Input: part model. Units: mm. Frame: model coordinates. Give positions to 0.01 mm unless a question says otherwise; leave off trailing zeros. Loops run counter-clockwise (first coordinate to the right, second up) from the corner with the lowest first, then second, coordinate; pieces in that order, holes last. Notation, with made-up numbers: M 67.25,60 L 111.25,60 A10 cw 111.25,64 Z; hole C -38.5,-6.75 d9. An arc over 180 degrees is marked long. Answer as a JSON object with one key per item and string values. Group by question number.
1) Section query C-C on z = 172.4. Return loops of the section in (x, y).
2) Section query A-A on z = -192.4. Return loops of the section in (x, y).
3) First-contact query: P1, Ø9.5, axis at y = -29.33, z = 172.4, coming from the +X side. Flat tip, straight axial feed; report the tip coordinate or a pass-through.
4) Section query B-B on x = 1. Return loops of the section in (y, z).
5) Ray query, L1, parallel to Z at x = 15.5, y = -36.75; L2, parallel to Z at x = 19, y = -33; L3, parallel to Z at x = 27.5, y = -24.5. Return the intervals inside material, ascending.
from build123d import *

# Parameters (mm, degrees)
SKETCH1_W           = 35
SKETCH1_H           = 30
BOSS_EXTRUDE1_DEPTH = 202.4
SKETCH4_R           = 6
CUT_EXTRUDE1_DEPTH  = 211.132863092
SKETCH5_R           = 6
CUT_EXTRUDE2_DEPTH  = 208.132591643
CHAMFER1_SIZE       = 0.3


with BuildPart() as part:
    # Sketch1 → Boss-Extrude1 (new, symmetric)
    with BuildSketch(Plane.XY):
        with Locations((14.720343273, -29.328998989)):
            Rectangle(SKETCH1_W, SKETCH1_H)
    extrude(amount=BOSS_EXTRUDE1_DEPTH, both=True)

    # Sketch4 → Cut-Extrude1 (cut, through all)
    with BuildSketch(Plane.ZY.offset(2.779656727)):
        with Locations(Location((172.4, -29.328998989, 0), (0, 0, 270))):
            Circle(SKETCH4_R)
        with Locations(Location((62.4, -29.328998989, 0), (0, 0, 270))):
            Circle(SKETCH4_R)
        with Locations(Location((117.4, -29.328998989, 0), (0, 0, 270))):
            Circle(SKETCH4_R)
    extrude(amount=-CUT_EXTRUDE1_DEPTH, mode=Mode.SUBTRACT)

    # Sketch5 → Cut-Extrude2 (cut, through all)
    with BuildSketch(Plane(origin=(0, -14.328998989, 0), x_dir=(1, 0, 0), z_dir=(0, 1, 0))):
        with Locations(Location((14.720343273, 192.4, 0), (0, 0, 270))):
            Circle(SKETCH5_R)
    extrude(amount=-CUT_EXTRUDE2_DEPTH, mode=Mode.SUBTRACT)

    # Chamfer1
    chamfer1_edges = [part.edges().sort_by_distance(p)[0] for p in [
        (32.220343273, -23.328998989, 172.4),
        (-2.779656727, -23.328998989, 172.4),
        (32.220343273, -23.328998989, 62.4),
        (-2.779656727, -23.328998989, 62.4),
        (32.220343273, -23.328998989, 117.4),
        (-2.779656727, -23.328998989, 117.4),
    ]]
    chamfer(chamfer1_edges, length=CHAMFER1_SIZE)


solid = part.part
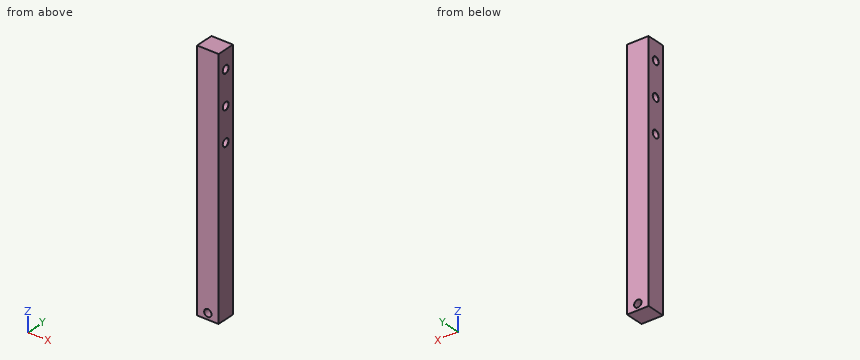
Output:
{
 "1": {"outline": "M -2.78,-44.33 L 32.22,-44.33 L 32.22,-35.63 L 31.92,-35.33 L -2.48,-35.33 L -2.78,-35.63 Z; M -2.78,-23.03 L -2.48,-23.33 L 31.92,-23.33 L 32.22,-23.03 L 32.22,-14.33 L -2.78,-14.33 Z"},
 "2": {"outline": "M -2.78,-44.33 L 8.72,-44.33 L 8.72,-14.33 L -2.78,-14.33 Z; M 20.72,-44.33 L 32.22,-44.33 L 32.22,-14.33 L 20.72,-14.33 Z"},
 "3": {"P1": "passes through"},
 "4": {"outline": "M -44.33,-202.4 L -14.33,-202.4 L -14.33,202.4 L -44.33,202.4 Z; hole C -29.33,62.4 d12; hole C -29.33,117.4 d12; hole C -29.33,172.4 d12"},
 "5": {"L1": "z = -202.4 to -198.35, -186.45 to 202.4", "L2": "z = -202.4 to -196.61, -188.19 to 57.65, 67.15 to 112.65, 122.15 to 167.65, 177.15 to 202.4", "L3": "z = -202.4 to 58.84, 65.96 to 113.84, 120.96 to 168.84, 175.96 to 202.4"}
}
